Part model, mm, in its own coordinate system. Face numbers are marked on the shaded views. A direction names the side the tool comes from. Round coordinates to 2 decimals unless told otherwise and drop trailing zeros. Loops run counter-clockwise (first coordinate to the right, second up) from the corner with the lowest first, then second, coordinate; pieces in that order, holes last. Notation, with made-up numbers: (50.5, -11.75) -> (74.5, -11.75) arc R32 cw to (74.5, 19.25) -> close; hole circle Ø9 at (74, 67). An arc over 180 degrees is marked (long way). Use a Markdown table: item, result. Add a question column.
Item 1: Flat gauge pins, fed straight in: pin 1 (2.5 mm diameter, centred on x = -5.5, z = 4, fed in from +Y); pin 2 (2 mm diameter, centred on x = 45, z = 4.5, fed in from -Y). Where does each tip first touch, or does it go through?
Item 2: Cut at B-B, the plane y = -11.5. State how many separate pieces and enclosed holes the cut face has, plus the area to 3 significant figures.
Item 3: Probe line 1 (X direction, y = -12, z = 3); line 2 (X direction, y = -6, z = 2); line 3 (X direction, y = -2.5, z = 28). List the from-to ranges inside material, lowest first. Write a range as [from, to].
Item 4: Which spindle directions (+Z, -Z, +X, -X, +Y, -Y) get a long thin tool onto all of the face, cutting with end or side? Do the marked faces 1, 2 and 3. Say none if no direction does.
Item 5: Cut at A-A, the plane z = 8.5. List the corners of the cut face in (x, y).
Item 6: Cut at C-C, the plane x = 43. List the corners of the cut face in (y, z).
```python
from build123d import *

# Parameters (mm, degrees)
SKETCH1_W                       = 42.960806382
SKETCH1_H                       = 31.115
BOSS_EXTRUDE1_DEPTH             = 12.7
SKETCH2_W                       = 42.960806382
SKETCH2_H                       = 22.225
BOSS_EXTRUDE2_DEPTH             = 19.05
BOSS_EXTRUDE3_DEPTH             = 22.225
DRAFT1_START                    = 15
DRAFT1_OUTLINE_W                = 22.225
DRAFT1_OUTLINE_H                = 19.270002336
DRAFT1_DEPTH                    = 6.752762537
BOSS_EXTRUDE4_REACH             = 69.308
SKETCH6_W                       = 42.960806382
SKETCH6_H                       = 4.445
DRAFT3_ANGLE                    = 20
DRAFT4_ANGLE                    = 20
BOSS_EXTRUDE5_DEPTH             = 22.225
F_6_CLEARANCE_HOLE1_D           = 4.3053
F_6_CLEARANCE_HOLE2_D           = 4.3053
F_6_CLEARANCE_HOLE2_ON_FACE_2_D = 4.3053
HOLE1_AT_2_COUNT                = 2
HOLE1_AT_2_PITCH                = 10.16
HOLE2_AT_2_COUNT                = 2
HOLE2_AT_2_PITCH                = 10.16
CUT_EXTRUDE1_DEPTH              = 70.758470007
CHAMFER1_SIZE                   = 2.54
CHAMFER2_SIZE                   = 0.762


with BuildPart() as part:
    # Sketch1 → Boss-Extrude1 (new body)
    with BuildSketch(Plane.XY):
        with Locations((1.668403191, -9.5885)):
            Rectangle(SKETCH1_W, SKETCH1_H)
    extrude(amount=BOSS_EXTRUDE1_DEPTH)

    # Sketch2 → Boss-Extrude2 (add)
    with BuildSketch(Plane.XY.offset(12.7)):
        with Locations((1.668403191, -9.5885)):
            Rectangle(SKETCH2_W, SKETCH2_H)
    extrude(amount=BOSS_EXTRUDE2_DEPTH)

    # Sketch3 → Boss-Extrude3 (add)
    with BuildSketch(Plane.XZ.offset(20.701)):
        Polygon((23.148806382, 31.75), (53.759077492, 31.75), (53.759077492, 0), (44.234077492, 0), (44.234077492, 18.107878998), (23.148806382, 18.107878998), align=None)
    extrude(amount=-BOSS_EXTRUDE3_DEPTH)

    # Draft1: read off the stored shape, not the designer's step
    # Draft1 outline → Draft1 (add)
    with BuildSketch(Plane(origin=(0, 0, 0), x_dir=(0, 1, 0), z_dir=(0.9396926207859083, 0, -0.3420201433256691)).offset(DRAFT1_START)):
        with Locations((-9.5885, 17.552359245)):
            Rectangle(DRAFT1_OUTLINE_W, DRAFT1_OUTLINE_H)
    extrude(amount=DRAFT1_DEPTH)

    # Sketch6 → Boss-Extrude4 (add, up to next)
    with BuildSketch(Plane.XY.offset(31.75), mode=Mode.PRIVATE) as boss_extrude4_sk1:
        with Locations((1.668403191, 3.7465)):
            Rectangle(SKETCH6_W, SKETCH6_H)
    boss_extrude4_tool1 = extrude(boss_extrude4_sk1.sketch, amount=-BOSS_EXTRUDE4_REACH, mode=Mode.PRIVATE) - part.part
    # Sketch6 → Boss-Extrude4 (add, up to next)
    with BuildSketch(Plane.XY.offset(31.75), mode=Mode.PRIVATE) as boss_extrude4_sk2:
        with Locations((1.668403191, -22.9235)):
            Rectangle(SKETCH6_W, SKETCH6_H)
    boss_extrude4_tool2 = extrude(boss_extrude4_sk2.sketch, amount=-BOSS_EXTRUDE4_REACH, mode=Mode.PRIVATE) - part.part
    add(boss_extrude4_tool1.solids().sort_by_distance((1.668403, 3.7465, 31.75))[0])
    add(boss_extrude4_tool2.solids().sort_by_distance((1.668403, -22.9235, 31.75))[0])

    # Draft3
    draft3_faces = [part.faces().sort_by_distance(p)[0] for p in [
        (23.148806382, -22.9235, 15.875),
    ]]
    draft(draft3_faces, Plane(origin=(23.148806382, -20.701, 31.75), x_dir=(-1, 0, 0), z_dir=(0, -1, 0)), DRAFT3_ANGLE)

    # Draft4
    draft4_faces = [part.faces().sort_by_distance(p)[0] for p in [
        (23.148806382, 3.7465, 15.875),
    ]]
    draft(draft4_faces, Plane(origin=(23.148806382, 1.524, 31.75), x_dir=(1, 0, 0), z_dir=(0, 1, 0)), DRAFT4_ANGLE)

    # Sketch8 → Boss-Extrude5 (add)
    with BuildSketch(Plane.XZ.offset(20.701)):
        Polygon((29.739535343, 18.107878998), (23.148806382, 0), (44.234077492, 0), (44.234077492, 18.107878998), align=None)
    extrude(amount=-BOSS_EXTRUDE5_DEPTH)

    # #6 Clearance Hole1 (through all)
    with Locations(Plane(origin=(0, -20.701, 0), x_dir=(-1, 0, 0), z_dir=(0, -1, 0))):
        with Locations((-48.996577492, -26.9875), (-48.996577492, -4.7625), (-29.498806382, -26.9875)):
            Hole(F_6_CLEARANCE_HOLE1_D / 2)

    # #6 Clearance Hole2 (through all)
    with Locations(Plane(origin=(-14.986, -25.146, 3.81), x_dir=(-1, 0, 0), z_dir=(0, -1, 0))):
        with Locations((0, 0), (-10.16, 0)):
            Hole(F_6_CLEARANCE_HOLE2_D / 2)

    # #6 Clearance Hole2 on face 2 (through all)
    with Locations(Plane(origin=(14.986, 5.969, 3.81), x_dir=(0, 0, 1), z_dir=(0, 1, 0))):
        with Locations((0, 0), (0, -10.16)):
            Hole(F_6_CLEARANCE_HOLE2_ON_FACE_2_D / 2)

    # Sketch18 → Hole1 (revolve, cut)
    with BuildSketch(Plane(origin=(-4.826, 5.969, 3.81), x_dir=(0, 0, 1), z_dir=(1, 0, 0))):
        Polygon((0, 0), (0, 3.81), (2.5273, 3.81), (2.6543, 0), align=None)
    hole1 = revolve(axis=Axis((-4.826, -104.031, 3.81), (0, 1, 0)), mode=Mode.SUBTRACT)

    # Hole1 at 2: Hole1 ×2
    with Locations(*[(-i * HOLE1_AT_2_PITCH, 0, 0) for i in range(1, HOLE1_AT_2_COUNT)]):
        add(hole1, mode=Mode.SUBTRACT)

    # Sketch20 → Hole2 (revolve, cut)
    with BuildSketch(Plane(origin=(4.826, -25.146, 3.81), x_dir=(0, 0, -1), z_dir=(1, 0, 0))):
        Polygon((0, 0), (0, 3.81), (2.5273, 3.81), (2.6543, 0), align=None)
    hole2 = revolve(axis=Axis((4.826, 84.854, 3.81), (0, -1, 0)), mode=Mode.SUBTRACT)

    # Hole2 at 2: Hole2 ×2
    with Locations(*[(i * HOLE2_AT_2_PITCH, 0, 0) for i in range(1, HOLE2_AT_2_COUNT)]):
        add(hole2, mode=Mode.SUBTRACT)

    # Sketch21 → Cut-Extrude1 (cut, through all)
    with BuildSketch(Plane(origin=(0, 5.969, 0), x_dir=(1, 0, 0), z_dir=(0, 1, 0))):
        Polygon((-19.812, -9.525), (-19.812, -31.75), (15.180958691, -31.75), align=None)
    extrude(amount=-CUT_EXTRUDE1_DEPTH, mode=Mode.SUBTRACT)

    # Chamfer1
    chamfer1_edges = [part.edges().sort_by_distance(p)[0] for p in [
        (53.759077492, -9.5885, 31.75),
        (53.759077492, -9.5885, 0),
    ]]
    chamfer(chamfer1_edges, length=CHAMFER1_SIZE)

    # Chamfer2
    chamfer2_edges = [part.edges().sort_by_distance(p)[0] for p in [
        (-19.812, -25.146, 4.7625),
        (-19.812, 5.969, 4.7625),
        (0.859479345, -25.146, 0),
        (-19.812, -9.5885, 0),
        (0.859479345, 5.969, 0),
    ]]
    chamfer(chamfer2_edges, length=CHAMFER2_SIZE)


solid = part.part
```
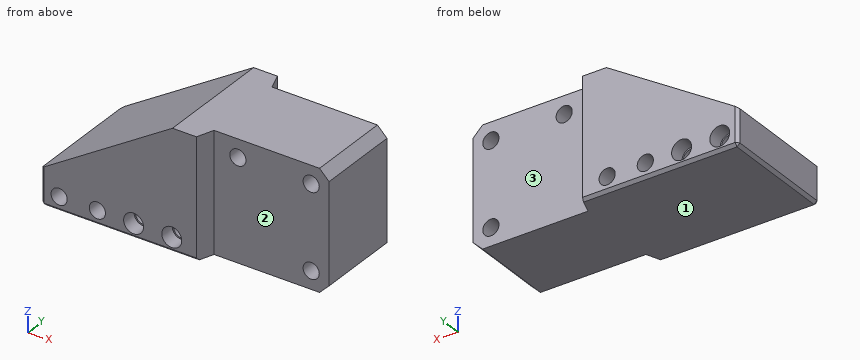
A:
| question | item | result |
|---|---|---|
| 1 | pin 1 | passes through |
| 1 | pin 2 | stops at y = -20.7 |
| 2 | separate pieces | 1 |
| 2 | enclosed holes | 7 |
| 2 | area | 1,840 mm^2 |
| 3 | line 1 | x = [-19.81, -16.98], [-12.99, -6.82], [-2.83, 2.83], [6.82, 12.99], [16.98, 47.76], [50.23, 53.76] |
| 3 | line 2 | x = [-19.81, -16.15], [-13.82, -5.99], [-3.66, 3.66], [5.99, 13.82], [16.15, 53.22] |
| 3 | line 3 | x = [9.28, 27.6], [31.4, 47.1], [50.9, 53.76] |
| 4 | face 1 | -Z, +X, -X, +Y, -Y |
| 4 | face 2 | +Z, -Z, +X, -Y |
| 4 | face 3 | +Z, -Z, +X, +Y |
| 5 | outline | (-19.81, -24.38) -> (-19.05, -25.15) -> (21.53, -25.15) -> (23.15, -20.7) -> (53.76, -20.7) -> (53.76, 1.52) -> (23.15, 1.52) -> (21.53, 5.97) -> (-19.05, 5.97) -> (-19.81, 5.21) -> close |
| 6 | outline | (-20.7, 0) -> (1.52, 0) -> (1.52, 31.75) -> (-20.7, 31.75) -> close |
